from build123d import *

# Parameters (mm, degrees)
BOSS_EXTRUDE1_DEPTH = 10
SKETCH2_W           = 10
SKETCH2_H           = 2
BOSS_EXTRUDE2_DEPTH = 38
SKETCH4_W           = 4
SKETCH4_H           = 38
BOSS_EXTRUDE3_DEPTH = 20
CUT_EXTRUDE1_REACH  = 43.355
SKETCH3_R           = 3.41


with BuildPart() as part:
    # Sketch1 → Boss-Extrude1 (new, symmetric)
    with BuildSketch(Plane.XY):
        Polygon((-2, 5), (2, 12.5), (2, -12.5), (-2, -12.5), align=None)
    extrude(amount=BOSS_EXTRUDE1_DEPTH, both=True)

    # Sketch2 → Boss-Extrude2 (add)
    with BuildSketch(Plane.XZ.offset(12.5)):
        with Locations((3, 11)):
            Rectangle(SKETCH2_W, SKETCH2_H)
        with Locations((3, -11)):
            Rectangle(SKETCH2_W, SKETCH2_H)
    extrude(amount=-BOSS_EXTRUDE2_DEPTH)

    # Sketch4 → Boss-Extrude3 (add)
    with BuildSketch(Plane(origin=(0, 0, -12), x_dir=(-1, 0, 0), z_dir=(0, 0, -1))):
        with Locations((0, 6.5)):
            Rectangle(SKETCH4_W, SKETCH4_H)
    extrude(amount=BOSS_EXTRUDE3_DEPTH)

    # Sketch3 → Cut-Extrude1 (cut, up to next)
    with BuildSketch(Plane(origin=(2, 0, 0), x_dir=(0, 0, -1), z_dir=(1, 0, 0)), mode=Mode.PRIVATE) as cut_extrude1_sk1:
        with Locations((22, -2.5)):
            Circle(SKETCH3_R)
    cut_extrude1_tool1 = extrude(cut_extrude1_sk1.sketch, amount=-CUT_EXTRUDE1_REACH, mode=Mode.PRIVATE) & part.part
    # Sketch3 → Cut-Extrude1 (cut, up to next)
    with BuildSketch(Plane(origin=(2, 0, 0), x_dir=(0, 0, -1), z_dir=(1, 0, 0)), mode=Mode.PRIVATE) as cut_extrude1_sk2:
        with Locations((22, 15.5)):
            Circle(SKETCH3_R)
    cut_extrude1_tool2 = extrude(cut_extrude1_sk2.sketch, amount=-CUT_EXTRUDE1_REACH, mode=Mode.PRIVATE) & part.part
    add(cut_extrude1_tool1.solids().sort_by_distance((2, -2.5, -22))[0], mode=Mode.SUBTRACT)
    add(cut_extrude1_tool2.solids().sort_by_distance((2, 15.5, -22))[0], mode=Mode.SUBTRACT)


solid = part.part
Here's how the part is built. I have some questions about the finished solid (model axes, mm). A direction names the side the tool comes from. Coordinates: 2 decimals unless noted, no trailing zeros. Order: outer loops, then holes, each group sorted by start corner. A loop starts at its lowest first (then second) coordinate and runs counter-clockwise, first axis right, second up. Notation, with made-up numbers: (30, 60.25) -> (72, 60.25) arc R31 ccw to (72, 99.25) -> close; hole circle Ø3 at (-38, -30). An arc over 180 degrees is marked (long way). Answer in a Markdown table with one row per item.
(1) I want a section at B-B on x = 6.5. List the corners of the cut face in (y, z) for me, then the cut area to 3 significant figures.
Answer key:
| item | result |
|---|---|
| outline | (-12.5, -12) -> (25.5, -12) -> (25.5, -10) -> (-12.5, -10) -> close; (-12.5, 10) -> (25.5, 10) -> (25.5, 12) -> (-12.5, 12) -> close |
| area | 152 mm^2 |
(2) I want a section at D-D on y = 15.5. List the corners of the cut face in (x, z) for me, then the cut area to 3 significant figures.
Answer key:
| item | result |
|---|---|
| outline | (-2, -32) -> (2, -32) -> (2, -25.41) -> (-2, -25.41) -> close; (-2, -18.59) -> (2, -18.59) -> (2, -12) -> (8, -12) -> (8, -10) -> (-2, -10) -> close; (-2, 10) -> (8, 10) -> (8, 12) -> (-2, 12) -> close |
| area | 92.7 mm^2 |
(3) On a 3-axis mill with a long thin cutter (end or side, diameter ignored), from which of +Z, -Z, +X, -X, +Y, -Y can I reach the whole of each face in a straight line? I mean faces 1 (the face through (2, 0, 0)), 2 (the face through (5, 6, -12)), 3 (the face through (3, 25.5, 11)). Say none if no direction works.
Answer key:
| item | result |
|---|---|
| face 1 | +X, +Y, -Y |
| face 2 | -Z, +X, +Y, -Y |
| face 3 | +Z, -Z, +X, -X, +Y |
(4) Will these pins go through, and if not, where does the flat tip stop? pin 1 Ø1 at (y, z) = (7, 3.5) entering from -X; pin 2 Ø22 at (y, z) = (0.5, -4.5) entering from +X; pin 3 Ø6 at (y, z) = (12, -18.5) entering from +X; pin 4 Ø5 at (x, y) = (5, 15) entering from -Z.
Answer key:
| item | result |
|---|---|
| pin 1 | x = -1.2 |
| pin 2 | x = 8 |
| pin 3 | x = 2 |
| pin 4 | z = -12 |
(5) Please list where these lines run through material, in increasing order: probe 1 along Y at (x, z) = (0.8, -22); probe 2 along Z at (x, y) = (6, -4); probe 3 along X at (y, z) = (1.5, -8.5).
Answer key:
| item | result |
|---|---|
| probe 1 | -12.5 to -5.91, 0.91 to 12.09, 18.91 to 25.5 |
| probe 2 | -12 to -10, 10 to 12 |
| probe 3 | -2 to 2 |
(6) Thinking about a two-plate mould opening in Z: for faces 4 (the face through (8, 6, 11)), 5 (the face through (3, 6, 12)), 6 (the face through (-0.028, 8.698, 0.14)), which applies, +Z half, -Z half, draft (parallel to the pull), parting line (faces both ways), or undercut?
Answer key:
| item | result |
|---|---|
| face 4 | draft |
| face 5 | +Z half |
| face 6 | undercut |
(7) I want a section at C-C on z = -22. List the corners of the cut face in (x, y) for me.
Answer key:
| item | result |
|---|---|
| outline | (-2, -12.5) -> (2, -12.5) -> (2, -5.91) -> (-2, -5.91) -> close; (-2, 0.91) -> (2, 0.91) -> (2, 12.09) -> (-2, 12.09) -> close; (-2, 18.91) -> (2, 18.91) -> (2, 25.5) -> (-2, 25.5) -> close |
(8) I want a section at A-A on y = -2.5. List the corners of the cut face in (x, z) for me.
Answer key:
| item | result |
|---|---|
| outline | (-2, -32) -> (2, -32) -> (2, -25.41) -> (-2, -25.41) -> close; (-2, -18.59) -> (2, -18.59) -> (2, -12) -> (8, -12) -> (8, -10) -> (2, -10) -> (2, 10) -> (8, 10) -> (8, 12) -> (-2, 12) -> close |
